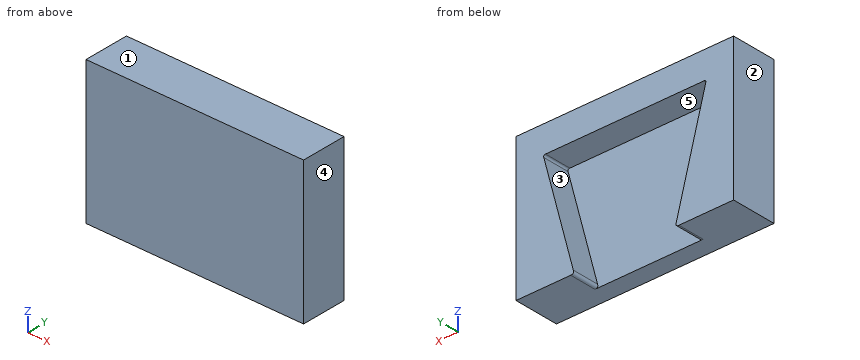
```python
from build123d import *

# Parameters (mm, degrees)
SKETCH1_W           = 24
SKETCH1_H           = 15.78
BOSS_EXTRUDE1_DEPTH = 5
CUT_EXTRUDE1_DEPTH  = 3


with BuildPart() as part:
    # Sketch1 → Boss-Extrude1 (new body)
    with BuildSketch(Plane(origin=(0, 0, 0), x_dir=(1, 0, 0), z_dir=(0, 1, 0))):
        with Locations((12, 7.89)):
            Rectangle(SKETCH1_W, SKETCH1_H)
    extrude(amount=BOSS_EXTRUDE1_DEPTH)

    # Sketch2 → Cut-Extrude1 (cut)
    with BuildSketch(Plane(origin=(0, 5, 0), x_dir=(1, 0, 0), z_dir=(0, 1, 0))):
        Polygon((6.424390679, 15.78), (3, 3), (21, 3), (17.575609321, 15.78), align=None)
    extrude(amount=-CUT_EXTRUDE1_DEPTH, mode=Mode.SUBTRACT)

    # Fillet1
    # a fillet whose section is not a circle: 0.2 mm, written as the material it adds along each edge
    with BuildSketch(Plane(origin=(21, 5, -3), x_dir=(-1, 0, 0), z_dir=(0, -1, 0)), Plane(origin=(3, 5, -3), x_dir=(0.25881904510252013, 0, -0.9659258262890685), z_dir=(0, -1, 0))) as fillet1_piece_1:
        with BuildLine():
            add(Edge.make_bspline([(0.260645075, 0), (0.21890515, 0), (0.177165225, 0), (0.086689828, 0.021204892), (0.042919331, 0.078247714), (0.045853734, 0.171128466), (0.056656822, 0.211446138), (0.067459909, 0.251763809)], knots=[0, 0, 0, 0, 0, 0, 0.5, 0.5, 1, 1, 1, 1, 1, 1], degree=5))
            Line((0.067459909, 0.251763809), (0, 0))
            Line((0, 0), (0.260645075, 0))
        make_face()
    extrude(amount=3.651612686)

    # Fillet2
    # a fillet whose section is not a circle: 0.3 mm, written as the material it takes off along each edge
    with BuildSketch(Plane(origin=(6.424390679, 5.97741903, -15.78), x_dir=(-1, 0, 0), z_dir=(0, -1, 0)), Plane(origin=(17.575609321, 5.97741903, -15.78), x_dir=(0.25881904510251846, 0, 0.9659258262890689), z_dir=(0, -1, 0))) as fillet2_piece_1:
        with BuildLine():
            add(Edge.make_bspline([(0.390967612, 0), (0.328357725, 0), (0.265747838, 0), (0.130034743, -0.031807338), (0.064378997, -0.117371571), (0.068780602, -0.2566927), (0.084985233, -0.317169207), (0.101189864, -0.377645714)], knots=[0, 0, 0, 0, 0, 0, 0.5, 0.5, 1, 1, 1, 1, 1, 1], degree=5))
            Line((0.101189864, -0.377645714), (0, 0))
            Line((0, 0), (0.390967612, 0))
        make_face()
    extrude(amount=3.97741903, mode=Mode.SUBTRACT)


solid = part.part
```
Build history of the part. All positions in model axes, mm. Face numbers are marked on the shaded views. A direction names the side the tool comes from. Round coordinates to 2 decimals unless told otherwise and drop trailing zeros. Loops run counter-clockwise (first coordinate to the right, second up) from the corner with the lowest first, then second, coordinate; pieces in that order, holes last.
Item 1: Saw through at A-A (x = 11). List the corners of the cut face in (y, z).
Item 2: Two-plate mould, pull along X, no slides. Class the marked faces 1, 2 and 3: released by +X, released by -X, zero draft, split by the parting line, or undercut.
Item 3: Drill centre lines: line 1 along Z through (x, y) = (13.5, 3.5); line 2 along Y through (x, z) = (18.25, -6.75); line 3 along X through (y, z) = (4.45, -9.5). Where is each one in solid material? Low to high.
Item 4: Pin check, flat tip, straight feed: P1, Ø6.5, axis at x = 10, z = -9.5, coming from the +Y side. Stop position of the tip, or through.
Item 5: Saw through at C-C (x = 5). List the corners of the cut face in (y, z), then the cut area to 3 significant figures.
Item 6: Saw through at B-B (z = -9). List the corners of the cut face in (x, y), then the cut area to 3 significant figures.
Item 7: Which spindle directions (+Z, -Z, +X, -X, +Y, -Y) get a long thin tool onto all of the face, cutting with end or side? Do the marked faces 4 and 5. Say none if no direction does.
Worked answers:
1. outline: (0, -15.78) - (2, -15.78) - (2, -3) - (5, -3) - (5, 0) - (0, 0) - close
2. face 1: zero draft
2. face 2: released by -X
2. face 3: undercut
3. line 1: z = -3 to 0
3. line 2: y = 0 to 2
3. line 3: x = 0 to 4.74, 19.26 to 24
4. P1: stops at y = 2
5. outline: (0, -15.78) - (5, -15.78) - (5, -10.46) - (2, -10.46) - (2, -3) - (5, -3) - (5, 0) - (0, 0) - close
5. area: 56.5 mm2
6. outline: (0, 0) - (24, 0) - (24, 5) - (19.39, 5) - (19.39, 2) - (4.61, 2) - (4.61, 5) - (0, 5) - close
6. area: 75.6 mm2
7. face 4: +Z, -Z, +X, +Y, -Y
7. face 5: +Y
